The model under review builds one solid part; all positions refer to its coordinate system, in mm. Give positions to 0.01 mm unless a question says otherwise; leave off trailing zeros. Order: outer loops, then holes, each group sorted by start corner. A loop starts at its lowest first (then second) coordinate and runs counter-clockwise, first axis right, second up. Notation, with made-up numbers: (-31, -21) -> (-16, -21) arc R8 cw to (-16, -13) -> close; hole circle Ø3 at (1, 45). An arc over 180 degrees is marked (long way). Use one line per item in the form item = value.
```python
from build123d import *

# Parameters (mm, degrees)
FILLET1_R    = 0.1
SKETCH3_W    = 0.74
SKETCH3_H    = 2.5
SKETCH4_W    = 0.74
SKETCH4_H    = 1.183744774
RECPAT_COUNT = 2
RECPAT_ANGLE = 90


with BuildPart() as part:
    # BodySke → Base-Revolve (revolve)
    with BuildSketch(Plane.XY):
        with BuildLine():
            Line((1.5, 1.25), (1.5, 2.65))
            Line((1.5, 2.65), (1.49, 2.65))
            Line((1.49, 2.65), (0.5, 2.563386223))
            ThreePointArc((0.5, 2.563386223), (0.126166852, 1.305847323), (0, 0))
            Line((0, 0), (6.5, 0))
            Line((6.5, 0), (6.5, 1.25))
            Line((6.5, 1.25), (1.5, 1.25))
        make_face()
    revolve(axis=Axis((-25.4, 0, 0), (1, 0, 0)))

    # Fillet1
    fillet1_edges = [part.edges().sort_by_distance(p)[0] for p in [
        (1.5, -1.25, 0),
    ]]
    fillet(fillet1_edges, radius=FILLET1_R)

    # Sketch3 → Recess section 0
    with BuildSketch(Plane(origin=(0, 0, 0), x_dir=(0, 0, -1), z_dir=(1, 0, 0))):
        Rectangle(SKETCH3_W, SKETCH3_H)
    # Sketch4 → Recess section 1
    with BuildSketch(Plane(origin=(1.32, 0, 0), x_dir=(0, 0, -1), z_dir=(1, 0, 0))):
        Rectangle(SKETCH4_W, SKETCH4_H)
    recess = loft(mode=Mode.SUBTRACT)

    # RecPat: Recess ×2 about axis
    recpat_axis = Axis((0, 0, 0), (1, 0, 0))
    for i in range(1, RECPAT_COUNT):
        add(recess.rotate(recpat_axis, i * RECPAT_ANGLE / (RECPAT_COUNT - 1)), mode=Mode.SUBTRACT)

    # RecCorSke → RecessCore (revolve, cut)
    with BuildSketch(Plane.XY):
        Polygon((0, 0), (0, 0.648303392), (1.32, 0.556), (1.500655351, 0), align=None)
    revolve(axis=Axis((-3.175, 0, 0), (1, 0, 0)), mode=Mode.SUBTRACT)


solid = part.part
```
1. The part is to be moulded in two halves that separate along Z. For faces 1 (the face through (6.5, 0, 0)), 2 (the face through (1.5, 0, 0)), 3 (the face through (0.77, 1.39, 2.18)), say which applies: +Z half, -Z half, draft (parallel to the pull), parting line (faces both ways), or undercut.
Values:
face_1 = draft
face_2 = undercut
face_3 = parting line
2. For pin 1 Ø1.5 at (x, y) = (1, 2) entering from -Z; pin 2 Ø3 at (x, z) = (4, -1.5) entering from -Y; pin 3 Ø1 at (x, y) = (1, -0.5) entering from -Z, all flat-tipped, find the tip position at first contact; note any pin that passes through.
Values:
pin_1 = -2.29
pin_2 = -1.25
pin_3 = -2.63
3. For L1, parallel to Y at x = 1.25, z = -0.2; L2, parallel to Z at x = 1, y = -0.25; L3, parallel to Z at x = 1, y = 0.5, list the stretches that pass through material, from the lowest coordinate up.
Values:
L1 = -2.62 to -0.63, 0.63 to 2.62
L2 = -2.6 to -0.75, 0.75 to 2.6
L3 = -2.56 to -0.37, 0.37 to 2.56
4. Add section A-A on x = 4.25. Give the boundary of the cut face in (y, z), then the cut area to 3 significant figures.
Values:
outline = circle Ø2.5 at (0, 0)
area = 4.91 mm^2
